from build123d import *

# Parameters (mm, degrees)
F0_W     = 145
F0_H     = 85
F1_DEPTH = 5
F2_W     = 6
F2_H     = 11
F2_H_2   = 5
F3_DEPTH = 5
F4_SIZE2 = 4.99999
F4_SIZE  = 1.99999


# Not quite as in the source:
# - a fillet or chamfer is up to 0.001 mm smaller than in the source, because OpenCascade refuses the exact size


with BuildPart() as f1:
    # F0 (on Front) → F1 (new body)
    with BuildSketch(Plane.XZ):
        Rectangle(F0_W, F0_H)
    extrude(amount=F1_DEPTH)

    # F2 (on Front) → F3 (cut, through all)
    with BuildSketch(Plane.XZ):
        with Locations((-36.25, 7)):
            Rectangle(F2_W, F2_H)
        with Locations((-48.25, -17)):
            Rectangle(F2_W, F2_H_2)
        with Locations((-24.25, -17)):
            Rectangle(F2_W, F2_H_2)
        with Locations((36.25, 7)):
            Rectangle(F2_W, F2_H)
        with Locations((48.25, -17)):
            Rectangle(F2_W, F2_H_2)
        with Locations((24.25, -17)):
            Rectangle(F2_W, F2_H_2)
    extrude(amount=F3_DEPTH, mode=Mode.SUBTRACT)

    # F4 (size 2 and 5 in the source; OpenCascade refuses exactly that, so slightly less here)
    f4_edges = [f1.edges().sort_by_distance(p)[0] for p in [
        (0, -5, 42.5),
        (-72.5, -5, 0),
        (0, -5, -42.5),
        (72.5, -5, 0),
    ]]
    f4_side = f1.faces().sort_by_distance((0, -5, 0.092438))[0]
    chamfer(f4_edges, length=F4_SIZE, length2=F4_SIZE2, reference=f4_side)


solid = f1.part
Verification items for the finished model (mm, model axes). A direction names the side the tool comes from. Coordinates: 2 decimals unless noted, no trailing zeros. Write each loop counter-clockwise with the first axis right and the second up, starting at its lowest first coordinate (ties: lowest second). Pieces come first, ordered by that corner, then holes. Notation, with made-up numbers: M 31,-36 L 60,-36 A32 ccw 60,3 Z; hole C 29.25,84 d6. An arc over 180 degrees is marked long. One line per question, with ' | ' between items.
1) Depth check by flat-ended pin: pin 1 Ø1.5 at (x, y) = (-49.5, -3) entering from -Z; pin 2 Ø1.5 at (x, y) = (-23, -2.5) entering from -Z; pin 3 Ø1.5 at (y, z) = (-4, -20.5) entering from -X; pin 4 Ø1.5 at (x, z) = (-11.5, -24) entering from +Y. Enter the tip coordinate at first touch or a pass-through.
Solutions:
pin 1: z = -41.6 | pin 2: z = -41.8 | pin 3: x = -71.2 | pin 4: y = 0
2) Material ranges on L1, parallel to X at y = -2.4, z = 10.5; L2, parallel to X at y = -0.2, z = 7; L3, parallel to Z at x = 46.5, y = -1.9, recorded low to high.
Solutions:
L1: -71.54 to -39.25, -33.25 to 33.25, 39.25 to 71.54 | L2: -72.42 to -39.25, -33.25 to 33.25, 39.25 to 72.42 | L3: -41.74 to -19.5, -14.5 to 41.74
3) Release check for a two-part mould opening along Z. For faces 3 (the face through (33.25, -2, 7)), 4 (the face through (71.5, -2.5, -0.6)), 5 (the face through (-1, -2.5, -41.5)) record: +Z half, -Z half, draft (parallel to the pull), parting line (faces both ways), or undercut.
Solutions:
face 3: undercut | face 4: draft | face 5: -Z half
4) Access from +Z, -Z, +X, -X, +Y, -Y to the whole of each face (thin tool, end or side, straight path). Record for faces 1 (the face through (-48, -2, -19.5)), 2 (the face through (-1, -2.5, 41.5)).
Solutions:
face 1: +Y, -Y | face 2: +Z, +X, -X, -Y
5) Sectioned sample at A-A on z = 10. State how many separate pieces and enclosed holes the cut face has, then the cut area to 3 significant figures.
Solutions:
separate pieces: 3 | enclosed holes: 0 | area: 655 mm^2
6) Sectioned sample at B-B on y = -2.4. Record the cut outline in (x, z), then the cut area to 3 significant figures.
Solutions:
outline: M -71.54,-41.54 L 71.54,-41.54 L 71.54,41.54 L -71.54,41.54 Z; hole M -51.25,-19.5 L -45.25,-19.5 L -45.25,-14.5 L -51.25,-14.5 Z; hole M -39.25,1.5 L -33.25,1.5 L -33.25,12.5 L -39.25,12.5 Z; hole M -27.25,-19.5 L -21.25,-19.5 L -21.25,-14.5 L -27.25,-14.5 Z; hole M 21.25,-19.5 L 27.25,-19.5 L 27.25,-14.5 L 21.25,-14.5 Z; hole M 33.25,1.5 L 39.25,1.5 L 39.25,12.5 L 33.25,12.5 Z; hole M 45.25,-19.5 L 51.25,-19.5 L 51.25,-14.5 L 45.25,-14.5 Z | area: 11,600 mm^2
